The figure shows three views and two pictorial views of one solid part (mm, origin at its lowest corner). Answer the questions. A direction names the side the tool comes from. Coordinates: 2 decimals unless noted, no trailing zeros. Write each loop counter-clockwise with the first axis right and the second up, starting at its lowest first coordinate (ties: lowest second). Pieces come first, ordered by that corner, then holes.
Item 1: Straight lines are drawn through the part: probe 1 along Y at (x, z) = (36.5, 19.6); probe 2 along Z at (x, y) = (33, 2.5); probe 3 along X at (y, z) = (36, 19). For each, find the intervals that lie inside material, in ascending order.
Item 2: Section D-D (x = 13) is taken. Give the vertices of the cut face in (y, z).
Item 3: Section C-C (z = 45) is taken. Give the vertices of the cut face in (x, y).
Item 4: A tool of negligible diameter and unlimited length cuts with its end or side. For the marked faces 1 and 2, from which of +Z, -Z, +X, -X, +Y, -Y can it reach the whole face along a straight path? Write none if from no direction.
Item 5: Section A-A (x = 21) is taken. Give the vertices of the cut face in (y, z), then the cut area to 4 significant figures.
Item 6: Each of these flat-tipped pins is pushed along its axis until it touches: P1, Ø10, axis at x = 15, z = 25, coming from the -Y side; P2, Ø12, axis at x = 8, y = 5.5, coming from the +Z side; P3, Ø10, axis at x = 13.5, y = 34, coming from the +Z side; P4, Ø6, axis at y = 14, z = 27, coming from the -X side. Where does it stop, or does it pass through?
Item 7: Section B-B (y = 5.5) is taken. Give the vertices of the cut face in (x, z).
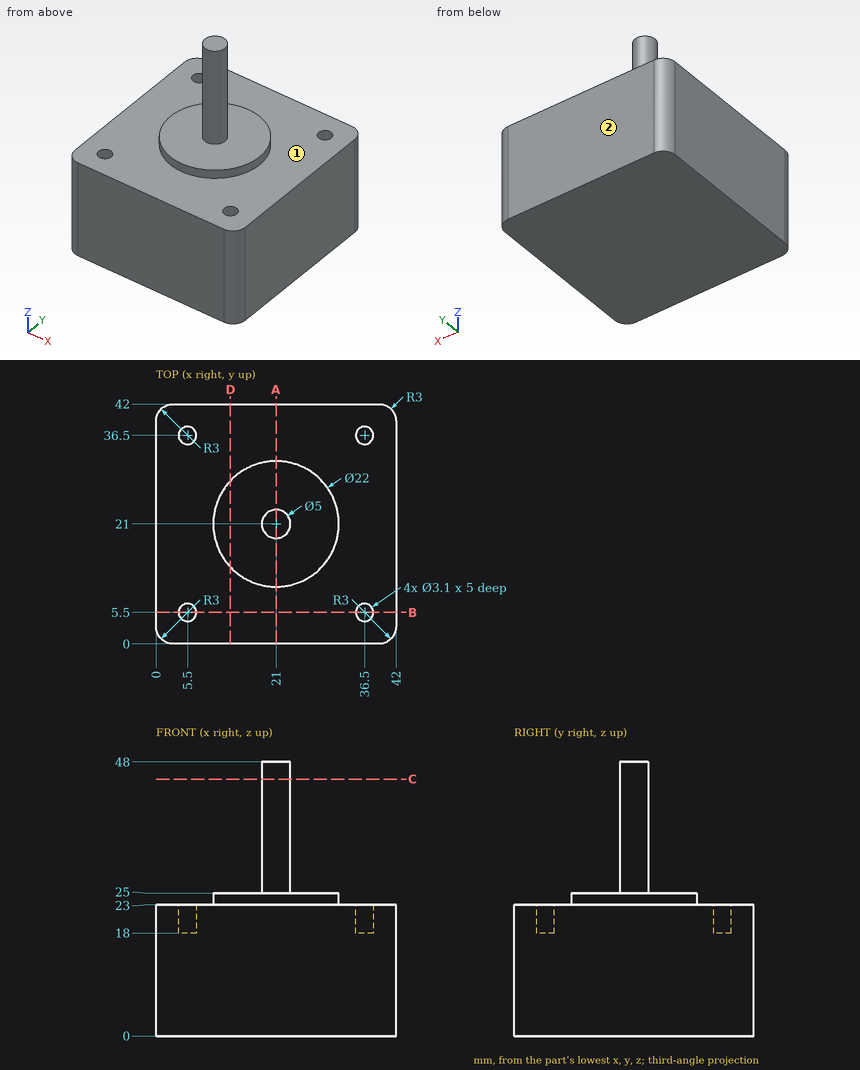
Established:
1. probe 1: y = 0 to 3.95, 7.05 to 34.95, 38.05 to 42
1. probe 2: z = 0 to 23
1. probe 3: x = 0 to 4.03, 6.97 to 35.03, 37.97 to 42
2. outline: (0, 0) - (42, 0) - (42, 23) - (28.55, 23) - (28.55, 25) - (13.45, 25) - (13.45, 23) - (0, 23) - close
3. outline: circle Ø5 at (21, 21)
4. face 1: +Z
4. face 2: +Z, -Z, +X, -X, +Y
5. outline: (0, 0) - (42, 0) - (42, 23) - (32, 23) - (32, 25) - (23.5, 25) - (23.5, 48) - (18.5, 48) - (18.5, 25) - (10, 25) - (10, 23) - (0, 23) - close
5. area: 1,125 mm2
6. P1: stops at y = 0
6. P2: stops at z = 23
6. P3: stops at z = 25
6. P4: stops at x = 11.09
7. outline: (0, 0) - (42, 0) - (42, 23) - (38.05, 23) - (38.05, 18) - (34.95, 18) - (34.95, 23) - (7.05, 23) - (7.05, 18) - (3.95, 18) - (3.95, 23) - (0, 23) - close
